Input: part model. Units: mm. Frame: model coordinates. Round coordinates to 2 decimals unless told otherwise and drop trailing zeros. Order: outer loops, then holes, each group sorted by start corner. A loop starts at its lowest first (then second) coordinate and runs counter-clockwise, first axis right, second up. Notation, with made-up numbers: (-19.75, 72) -> (-0.75, 72) arc R32 cw to (-0.75, 101) -> close; hole circle Ø4 at (2, 5). An arc over 180 degrees is marked (long way). Use a Markdown table: item, result.
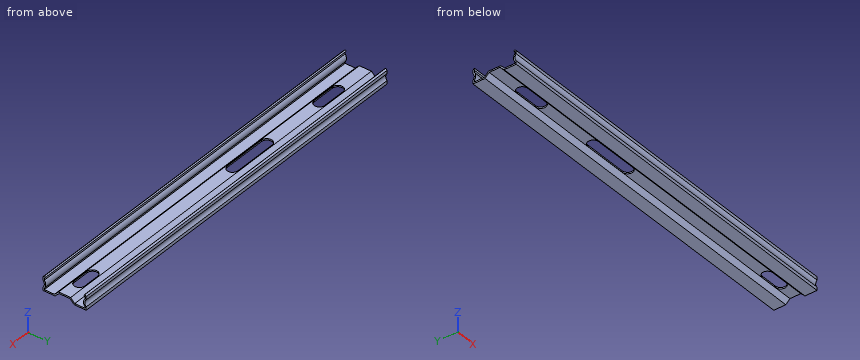
from build123d import *

# Parameters (mm, degrees)
EXTRUDE_THIN1_DEPTH   = 282
CORTE_EXTRUS_O1_DEPTH = 283.522008592


with BuildPart() as part:
    # Sketch1 → Extrude-Thin1 (new body)
    with BuildSketch(Plane(origin=(0, 0, 0), x_dir=(0, 0, -1), z_dir=(1, 0, 0))):
        with BuildLine():
            Line((-12.7, 14.804915028), (-11.7, 15.804915028))
            Line((-11.7, 15.804915028), (-9.401071342, 15.804915028))
            ThreePointArc((-9.401071342, 15.804915028), (-6.901071342, 14.85), (-4.401071342, 15.804915028))
            Line((-4.401071342, 15.804915028), (-2, 15.804915028))
            Line((-2, 15.804915028), (-2, 7))
            Line((-2, 7), (-5, 4))
            Line((-5, 4), (-5, -4))
            Line((-5, -4), (-2, -7))
            Line((-2, -7), (-2, -15.804915028))
            Line((-2, -15.804915028), (-4.401071342, -15.804915028))
            ThreePointArc((-4.401071342, -15.804915028), (-6.901071342, -14.85), (-9.401071342, -15.804915028))
            Line((-9.401071342, -15.804915028), (-11.7, -15.804915028))
            Line((-11.7, -15.804915028), (-12.7, -14.804915028))
            Line((-12.7, -14.804915028), (-11.992893219, -14.097808247))
            Line((-11.992893219, -14.097808247), (-11.285786438, -14.804915028))
            Line((-11.285786438, -14.804915028), (-9.757612967, -14.804915028))
            ThreePointArc((-9.757612967, -14.804915028), (-6.901071342, -13.85), (-4.044529716, -14.804915028))
            Line((-4.044529716, -14.804915028), (-3, -14.804915028))
            Line((-3, -14.804915028), (-3, -7.414213562))
            Line((-3, -7.414213562), (-6, -4.414213562))
            Line((-6, -4.414213562), (-6, 4.414213562))
            Line((-6, 4.414213562), (-3, 7.414213562))
            Line((-3, 7.414213562), (-3, 14.804915028))
            Line((-3, 14.804915028), (-4.044529716, 14.804915028))
            ThreePointArc((-4.044529716, 14.804915028), (-6.901071342, 13.85), (-9.757612967, 14.804915028))
            Line((-9.757612967, 14.804915028), (-11.285786438, 14.804915028))
            Line((-11.285786438, 14.804915028), (-11.992893219, 14.097808247))
            Line((-11.992893219, 14.097808247), (-12.7, 14.804915028))
        make_face()
    extrude(amount=-EXTRUDE_THIN1_DEPTH)

    # Esboço1 → Corte-extrusão1 (cut, through all)
    with BuildSketch(Plane.XY.offset(6)):
        with BuildLine():
            Line((-13.9, -3.9), (-26.1, -3.9))
            ThreePointArc((-26.1, -3.9), (-30, 0), (-26.1, 3.9))
            Line((-26.1, 3.9), (-13.9, 3.9))
            ThreePointArc((-13.9, 3.9), (-10, 0), (-13.9, -3.9))
        make_face()
        with BuildLine():
            Line((-189.6, 3.9), (-157.4, 3.9))
            ThreePointArc((-157.4, 3.9), (-153.5, 0), (-157.4, -3.9))
            Line((-157.4, -3.9), (-189.6, -3.9))
            ThreePointArc((-189.6, -3.9), (-193.5, 0), (-189.6, 3.9))
        make_face()
        with BuildLine():
            Line((-256.1, 3.9), (-238.9, 3.9))
            ThreePointArc((-238.9, 3.9), (-235, 0), (-238.9, -3.9))
            Line((-238.9, -3.9), (-256.1, -3.9))
            ThreePointArc((-256.1, -3.9), (-260, 0), (-256.1, 3.9))
        make_face()
    extrude(amount=-CORTE_EXTRUS_O1_DEPTH, mode=Mode.SUBTRACT)


solid = part.part
1) Cut plane C-C on x = -63. Return loops of the section in (y, z), and give its area (3 significant figures).
Results found:
| item | result |
|---|---|
| outline | (-15.8, 2) -> (-7, 2) -> (-4, 5) -> (4, 5) -> (7, 2) -> (15.8, 2) -> (15.8, 4.4) arc R3.75 cw to (15.8, 9.4) -> (15.8, 11.7) -> (14.8, 12.7) -> (14.1, 11.99) -> (14.8, 11.29) -> (14.8, 9.76) arc R4.75 ccw to (14.8, 4.04) -> (14.8, 3) -> (7.41, 3) -> (4.41, 6) -> (-4.41, 6) -> (-7.41, 3) -> (-14.8, 3) -> (-14.8, 4.04) arc R4.75 ccw to (-14.8, 9.76) -> (-14.8, 11.29) -> (-14.1, 11.99) -> (-14.8, 12.7) -> (-15.8, 11.7) -> (-15.8, 9.4) arc R3.75 cw to (-15.8, 4.4) -> close |
| area | 54.4 mm² |
2) Line query: L1, parallel to Y at x = -26, z = 7; L2, parallel to Z at x = -18.5, y = 14.5; L3, parallel to Y at x = -152, z = 4.25. Output: solid intervals per line, ascending. Write a range as [from, to].
Results found:
| item | result |
|---|---|
| L1 | y = [-14.85, -13.85], [13.85, 14.85] |
| L2 | z = [2, 3], [4.5, 9.3], [11.59, 12.4] |
| L3 | y = [-15.8, -14.66], [-6.16, -4.75], [4.75, 6.16], [14.66, 15.8] |
3) Cut plane D-D on y = 11. Return loops of the section in (x, z).
Results found:
| item | result |
|---|---|
| outline | (-282, 2) -> (0, 2) -> (0, 3) -> (-282, 3) -> close |
4) Cut plane B-B on y = 1. Return loops of the section in (x, z), and give its area (3 significant figures).
Results found:
| item | result |
|---|---|
| outline | (-282, 5) -> (-259.87, 5) -> (-259.87, 6) -> (-282, 6) -> close; (-235.13, 5) -> (-193.37, 5) -> (-193.37, 6) -> (-235.13, 6) -> close; (-153.63, 5) -> (-29.87, 5) -> (-29.87, 6) -> (-153.63, 6) -> close; (-10.13, 5) -> (0, 5) -> (0, 6) -> (-10.13, 6) -> close |
| area | 198 mm² |
5) Pin query (flat end, axial travel): pin 1 Ø3.5 at (x, y) = (-75.5, 12) entering from +Z; pin 2 Ø0.8 at (x, z) = (-179, 5.5) entering from -Y; pin 3 Ø6 at (y, z) = (1, 7.5) entering from +X; pin 4 Ø3 at (x, z) = (-74.5, 7.5) entering from +Y. Return the tip coordinate at first contact, or that it passes through.
Results found:
| item | result |
|---|---|
| pin 1 | stops at z = 3 |
| pin 2 | stops at y = -15.31 |
| pin 3 | stops at x = 0 |
| pin 4 | stops at y = 15.49 |
